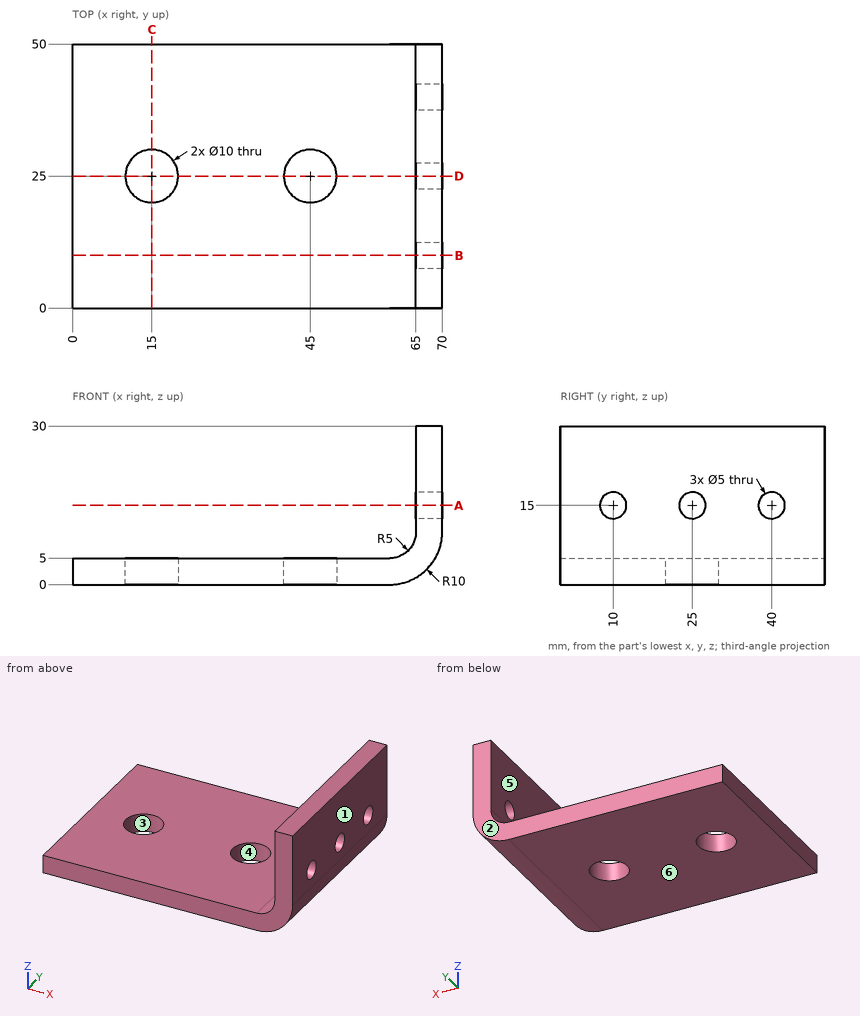
Job drawing, mm, ordinate dimensions from the low corner. One solid piece. A direction names the side the tool comes from. Coordinates: 2 decimals unless noted, no trailing zeros. Order: outer loops, then holes, each group sorted by start corner. A loop starts at its lowest first (then second) coordinate and runs counter-clockwise, first axis right, second up. Notation, with made-up numbers: (32, 9) -> (82, 9) arc R19 ccw to (82, 37) -> close; hole circle Ø4 at (45, -19.5). An arc over 180 degrees is marked (long way). Answer in a Markdown table with one row per item. Add a question column.
Q1. Wall check: line 1 along X through (y, z) = (28, 19.25); line 2 along Z through (x, y) = (24.5, 23); line 3 along Z through (x, y) = (68.75, 10). Give the ranges that are in metal, low to high. Write a range as [from, to].
Q2. Mould opens along X. For the marked faces 1, 2, 3 and 4 say: +X half, -X half, draft (parallel to the pull), parting line (faces both ways), or undercut.
Q3. Band-saw the part on C-C, the plane x = 15. List the corners of the cut face in (y, z), then the cut area to 3 significant figures.
Q4. Which spindle directions (+Z, -Z, +X, -X, +Y, -Y) get a long thin tool onto all of the face, cutting with end or side? Do the marked faces 5 and 6. Say none if no direction does.
Q5. Drop flat-ended pins along their axis: pin 1 (25 mm diameter, centred on x = 33.5, y = 30.5, fed in from +Z); pin 2 (3 mm diameter, centred on y = 10, z = 15, fed in from +X); pin 3 (16 mm diameter, centred on y = 29, z = 15.5, fed in from -X); pin 4 (6 mm diameter, centred on y = 25, z = 15, fed in from -X). Give the stop position or say it passes through.
Q6. Band-saw the part on D-D, the plane y = 25. List the corners of the cut face in (x, z), then the cut area to 3 significant figures.
Q7. Band-saw the part on B-B, the plane y = 10. List the corners of the cut face in (x, z), then the cut area to 3 significant figures.
Q8. Band-saw the part on A-A, the plane z = 15. List the corners of the cut face in (x, y).
Answers follow:
| question | item | result |
|---|---|---|
| 1 | line 1 | [65, 70] |
| 1 | line 2 | [0, 5] |
| 1 | line 3 | [5.16, 12.5], [17.5, 30] |
| 2 | face 1 | +X half |
| 2 | face 2 | draft |
| 2 | face 3 | undercut |
| 2 | face 4 | undercut |
| 3 | outline | (0, 0) -> (20, 0) -> (20, 5) -> (0, 5) -> close; (30, 0) -> (50, 0) -> (50, 5) -> (30, 5) -> close |
| 3 | area | 200 mm^2 |
| 4 | face 5 | +Z, -X, +Y, -Y |
| 4 | face 6 | -Z, +X, -X, +Y, -Y |
| 5 | pin 1 | z = 5 |
| 5 | pin 2 | through |
| 5 | pin 3 | x = 64.33 |
| 5 | pin 4 | x = 65 |
| 6 | outline | (0, 0) -> (10, 0) -> (10, 5) -> (0, 5) -> close; (20, 0) -> (40, 0) -> (40, 5) -> (20, 5) -> close; (50, 0) -> (60, 0) arc R10 ccw to (70, 10) -> (70, 12.5) -> (65, 12.5) -> (65, 10) arc R5 cw to (60, 5) -> (50, 5) -> close; (65, 17.5) -> (70, 17.5) -> (70, 30) -> (65, 30) -> close |
| 6 | area | 334 mm^2 |
| 7 | outline | (0, 0) -> (60, 0) arc R10 ccw to (70, 10) -> (70, 12.5) -> (65, 12.5) -> (65, 10) arc R5 cw to (60, 5) -> (0, 5) -> close; (65, 17.5) -> (70, 17.5) -> (70, 30) -> (65, 30) -> close |
| 7 | area | 434 mm^2 |
| 8 | outline | (65, 0) -> (70, 0) -> (70, 7.5) -> (65, 7.5) -> close; (65, 12.5) -> (70, 12.5) -> (70, 22.5) -> (65, 22.5) -> close; (65, 27.5) -> (70, 27.5) -> (70, 37.5) -> (65, 37.5) -> close; (65, 42.5) -> (70, 42.5) -> (70, 50) -> (65, 50) -> close |
